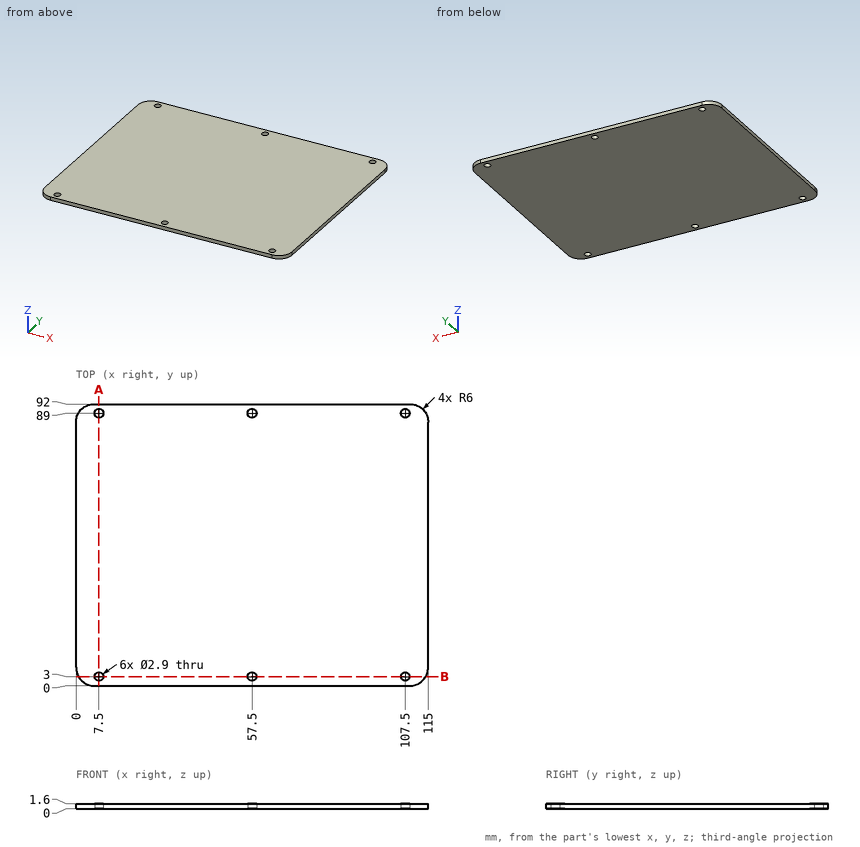
The drawing under review shows one solid part. Ordinate dimensions are in mm from its lowest x, y, z. Coordinates: 2 decimals unless noted, no trailing zeros. Order: outer loops, then holes, each group sorted by start corner. A loop starts at its lowest first (then second) coordinate and runs counter-clockwise, first axis right, second up. Notation, with made-up numbers: (18.25, 40.5) -> (57.25, 40.5) arc R30 ccw to (57.25, 63.5) -> close; hole circle Ø9 at (73, -0.5). An arc over 180 degrees is marked (long way). One line per item, written item: value.
1) We need section B-B, the plane y = 3. Give the boundary of the cut face in (x, z).
Output values:
outline: (0.8, 0) -> (6.05, 0) -> (6.05, 1.6) -> (0.8, 1.6) -> close; (8.95, 0) -> (56.05, 0) -> (56.05, 1.6) -> (8.95, 1.6) -> close; (58.95, 0) -> (106.05, 0) -> (106.05, 1.6) -> (58.95, 1.6) -> close; (108.95, 0) -> (114.2, 0) -> (114.2, 1.6) -> (108.95, 1.6) -> close
2) To check wall thickness, follow probe 1 along Y at (x, z) = (107.5, 0.6); probe 2 along X at (y, z) = (89, 0.6); probe 3 along Y at (x, z) = (8.5, 1.1). State the ranges of each line that lie inside material, in increasing order. Write a range as [from, to].
Output values:
probe 1: y = [0, 1.55], [4.45, 87.55], [90.45, 92]
probe 2: x = [0.8, 6.05], [8.95, 56.05], [58.95, 106.05], [108.95, 114.2]
probe 3: y = [0, 1.95], [4.05, 87.95], [90.05, 92]
3) We need section A-A, the plane x = 7.5. Give the boundary of the cut face in (y, z), then the cut area to 3 significant figures.
Output values:
outline: (0, 0) -> (1.55, 0) -> (1.55, 1.6) -> (0, 1.6) -> close; (4.45, 0) -> (87.55, 0) -> (87.55, 1.6) -> (4.45, 1.6) -> close; (90.45, 0) -> (92, 0) -> (92, 1.6) -> (90.45, 1.6) -> close
area: 138 mm2
